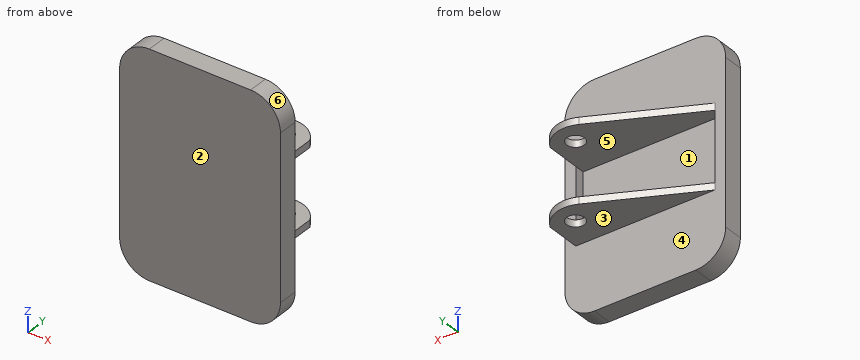
from build123d import *

# Parameters (mm, degrees)
EXTRUDE_1_DEPTH     = 10
SKETCH_2_W          = 70
SKETCH_2_H          = 42
EXTRUDE_2_DEPTH     = 27
SKETCH_3_W          = 70
SKETCH_3_H          = 35
CUT_EXTRUDE_1_DEPTH = 32
SKETCH_4_R          = 4.5
CUT_EXTRUDE_2_DEPTH = 118.724254086


with BuildPart() as part:
    # Sketch 150 → 凸台-拉伸1 (new body)
    with BuildSketch(Plane(origin=(0, 0, 0), x_dir=(1, 0, 0), z_dir=(0, 1, 0))):
        with BuildLine():
            Line((15, 0), (66, 0))
            ThreePointArc((66, 0), (76.606601718, 4.393398282), (81, 15))
            Line((81, 15), (81, 97))
            ThreePointArc((81, 97), (76.606601718, 107.606601718), (66, 112))
            Line((66, 112), (15, 112))
            ThreePointArc((15, 112), (4.393398282, 107.606601718), (0, 97))
            Line((0, 97), (0, 15))
            ThreePointArc((0, 15), (4.393398282, 4.393398282), (15, 0))
        make_face()
    extrude(amount=EXTRUDE_1_DEPTH)

    # 草图2 → 凸台-拉伸2 (add)
    with BuildSketch(Plane(origin=(0, 10, 0), x_dir=(1, 0, 0), z_dir=(0, 1, 0))):
        with Locations((40.5, 56)):
            Rectangle(SKETCH_2_W, SKETCH_2_H)
    extrude(amount=EXTRUDE_2_DEPTH)

    # 草图3 → 切除-拉伸1 (cut)
    with BuildSketch(Plane(origin=(0, 37, 0), x_dir=(1, 0, 0), z_dir=(0, 1, 0))):
        with Locations((40.5, 56)):
            Rectangle(SKETCH_3_W, SKETCH_3_H)
    extrude(amount=-CUT_EXTRUDE_1_DEPTH, mode=Mode.SUBTRACT)

    # 草图4 → 切除-拉伸2 (cut, through all)
    with BuildSketch(Plane.XY.offset(-35)):
        with Locations((64.5, 25)):
            Circle(SKETCH_4_R)
        with BuildLine():
            Line((5.5, 10), (2.465175939, 10))
            Line((2.465175939, 10), (2.465175939, 42.34627873))
            Line((2.465175939, 42.34627873), (79.036091511, 42.34627873))
            Line((79.036091511, 42.34627873), (79.036091511, 27.396377445))
            Line((79.036091511, 27.396377445), (75.5, 27.396377445))
            ThreePointArc((75.5, 27.396377445), (67.105558918, 34.896122118), (55.866672389, 34.26347622))
            Line((55.866672389, 34.26347622), (5.5, 10))
        make_face()
    extrude(amount=-CUT_EXTRUDE_2_DEPTH, mode=Mode.SUBTRACT)


solid = part.part
Could you check a few things on this model? Use its own coordinates, in mm. Face numbers are marked on the shaded views. A direction names the side the tool comes from. Give positions to 0.01 mm unless a question says otherwise; leave off trailing zeros. Write each loop counter-clockwise with the first axis right and the second up, starting at its lowest first coordinate (ties: lowest second). Pieces come first, ordered by that corner, then holes. Notation, with made-up numbers: (45, 8) -> (58, 8) arc R28 cw to (58, 29) -> close; hole circle Ø7 at (-31.75, 28). An arc over 180 degrees is marked (long way). Answer as a JSON object with one key per item and string values.
Q1. Suppose I cut it at D-D on z = -51. Write out the boundary of the cut face in (x, y).
Taken from the geometry:
{"outline": "(0, 0) -> (81, 0) -> (81, 10) -> (75.5, 10) -> (75.5, 5) -> (5.5, 5) -> (5.5, 10) -> (0, 10) -> close"}
Q2. Suppose I cut it at C-C on y = 14. Write out the boundary of the cut face in (x, z), then the cut area to 3 significant figures.
Taken from the geometry:
{"outline": "(13.8, -77) -> (75.5, -77) -> (75.5, -73.5) -> (13.8, -73.5) -> close; (13.8, -38.5) -> (75.5, -38.5) -> (75.5, -35) -> (13.8, -35) -> close", "area": "432 mm²"}
Q3. We'd pull the mould along Z, two halves only. Please class the marked faces 4, 5 and 6: released by +Z, released by -Z, zero draft, split by the parting line, or undercut.
Taken from the geometry:
{"face 4": "zero draft", "face 5": "undercut", "face 6": "released by +Z"}
Q4. Suppose I cut it at A-A on x = 64.5. Write out the boundary of the cut face in (y, z), then the cut area to 3 significant figures.
Taken from the geometry:
{"outline": "(0, -112) -> (10, -112) -> (10, -77) -> (20.5, -77) -> (20.5, -73.5) -> (5, -73.5) -> (5, -38.5) -> (20.5, -38.5) -> (20.5, -35) -> (10, -35) -> (10, 0) -> (0, 0) -> close; (29.5, -77) -> (35.55, -77) -> (35.55, -73.5) -> (29.5, -73.5) -> close; (29.5, -38.5) -> (35.55, -38.5) -> (35.55, -35) -> (29.5, -35) -> close", "area": "1,060 mm²"}
Q5. Which directions (+Z, -Z, +X, -X, +Y, -Y) give clear straight access to the entire face, cutting with the end or side of a thin tool? Please do the marked faces 1, 2 and 3.
Taken from the geometry:
{"face 1": "+Y", "face 2": "+Z, -Z, +X, -X, -Y", "face 3": "-Z, +X, -X, +Y"}
Q6. Suppose I cut it at B-B on z = -36.5. Write out the boundary of the cut face in (x, y).
Taken from the geometry:
{"outline": "(0, 0) -> (81, 0) -> (81, 10) -> (75.5, 10) -> (75.5, 27.4) arc R14.71 ccw to (55.87, 34.26) -> (5.5, 10) -> (0, 10) -> close; hole circle Ø9 at (64.5, 25)"}
Q7. Please list where these lines run through material, in increasing order: L1, parallel to Z at x = 36, y = 24; L2, parallel to Z at x = 62, y = 8.5; L3, parallel to Y at x = 64.5, z = -36.05.
Taken from the geometry:
{"L1": "z = -77 to -73.5, -38.5 to -35", "L2": "z = -112 to -73.5, -38.5 to 0", "L3": "y = 0 to 20.5, 29.5 to 35.55"}
Q8. Will these pins go through, and if not, where does the flat tip stop? pin 1 Ø15.5 at (x, y) = (51.5, 21.5) entering from +Z; pin 2 Ø4 at (x, z) = (30.5, -66.5) entering from +Y; pin 3 Ø2 at (x, z) = (28.5, -81.5) entering from -Y; pin 4 Ø9 at (x, y) = (50, 15) entering from -Z.
Taken from the geometry:
{"pin 1": "stops at z = -35", "pin 2": "stops at y = 5", "pin 3": "stops at y = 0", "pin 4": "stops at z = -77"}
